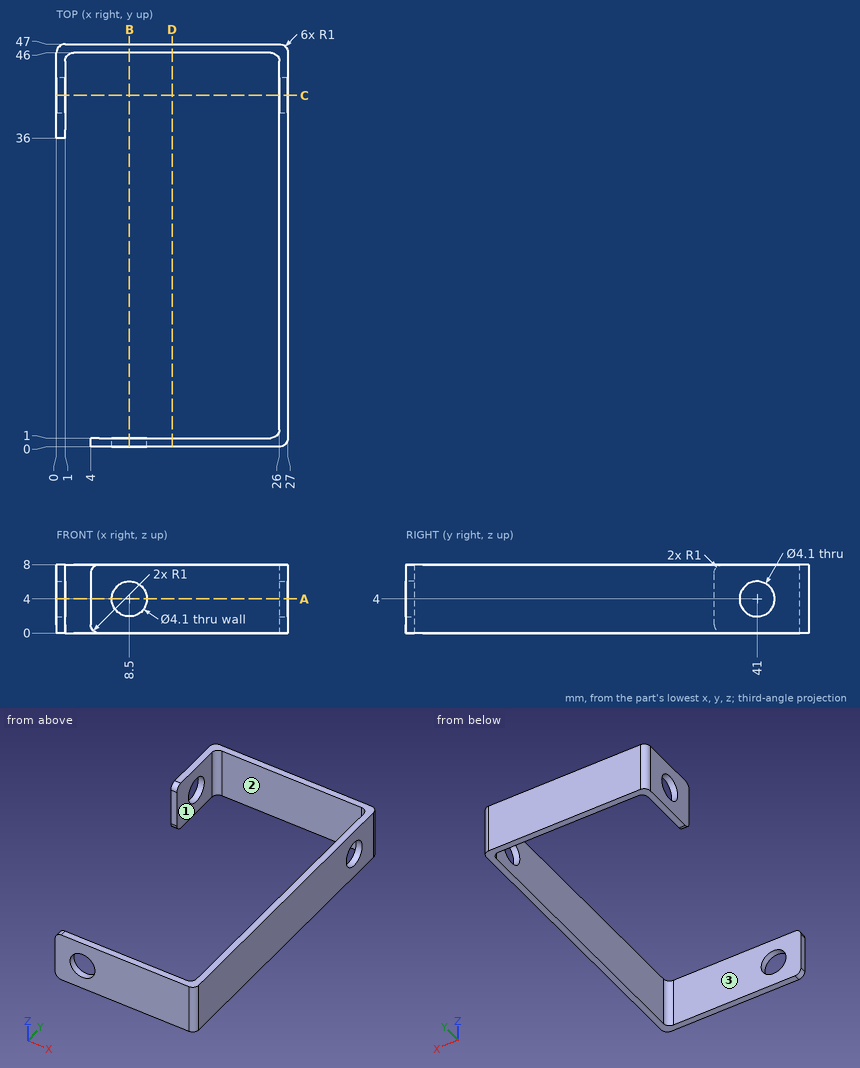
Verification items for this drawing (mm, ordinates from the low corner). A direction names the side the tool comes from. Give positions to 0.01 mm unless a question says otherwise; leave off trailing zeros. Loops run counter-clockwise (first coordinate to the right, second up) from the corner with the lowest first, then second, coordinate; pieces in that order, holes last. Notation, with made-up numbers: M 88,5.5 L 92,5.5 A29 cw 92,40.5 Z; hole C 46,74.5 d9. An arc over 180 degrees is marked long. Write item = value, one per line.
(1) Sectioned sample at B-B, the plane x = 8.5. Record the cut outline in (y, z), plus the area to 3 significant figures.
Answer below:
outline = M 0,0 L 1,0 L 1,1.95 L 0,1.95 Z; M 0,6.05 L 1,6.05 L 1,8 L 0,8 Z; M 46,0 L 47,0 L 47,8 L 46,8 Z
area = 11.9 mm2
(2) Sectioned sample at A-A, the plane z = 4. Record the cut outline in (x, y).
Answer below:
outline = M 0,36 L 1,36 L 1,38.95 L 0,38.95 Z; M 0,43.05 L 1,43.05 L 1,45 A1 cw 2,46 L 25,46 A1 cw 26,45 L 26,43.05 L 27,43.05 L 27,46 A1 ccw 26,47 L 1,47 A1 ccw 0,46 Z; M 4,0 L 6.45,0 L 6.45,1 L 4,1 Z; M 10.55,0 L 26,0 A1 ccw 27,1 L 27,38.95 L 26,38.95 L 26,2 A1 cw 25,1 L 10.55,1 Z
(3) Sectioned sample at C-C, the plane y = 41. Record the cut outline in (x, z), plus the area to 3 significant figures.
Answer below:
outline = M 0,0 L 1,0 L 1,1.95 L 0,1.95 Z; M 0,6.05 L 1,6.05 L 1,8 L 0,8 Z; M 26,0 L 27,0 L 27,1.95 L 26,1.95 Z; M 26,6.05 L 27,6.05 L 27,8 L 26,8 Z
area = 7.80 mm2
(4) Sectioned sample at D-D, the plane x = 13.5. Record the cut outline in (y, z).
Answer below:
outline = M 0,0 L 1,0 L 1,8 L 0,8 Z; M 46,0 L 47,0 L 47,8 L 46,8 Z
(5) Tool access check on the marked faces 1, 2 and 3. Record the directions out of +Z, -Z, +X, -X, +Y, -Y that give a thin tool (end or side, any length) a straight path to the whole face; none if there is none.
Answer below:
face_1 = +Z, -Z, -Y
face_2 = +Z, -Z
face_3 = +Z, -Z, -X
(6) Gauge pin test, flat ends, axial feed: pin 1 Ø3.5 at (x, z) = (8.5, 4) entering from -Y; pin 2 Ø2.5 at (y, z) = (25.5, 3) entering from -X; pin 3 Ø1.1 at (y, z) = (0.5, 3) entering from -X. Record the tip position at first contact, or that the pin passes through.
Answer below:
pin_1 = 46
pin_2 = 26
pin_3 = 4
(7) Material ranges on line 1 (Y direction, x = 20, z = 6.5); line 2 (Z direction, x = 26.5, y = 41); line 3 (X direction, y = 40, z = 2), recorded low to high. Write a range as [from, to].
Answer below:
line_1 = [0, 1], [46, 47]
line_2 = [0, 1.95], [6.05, 8]
line_3 = [0, 1], [26, 27]
